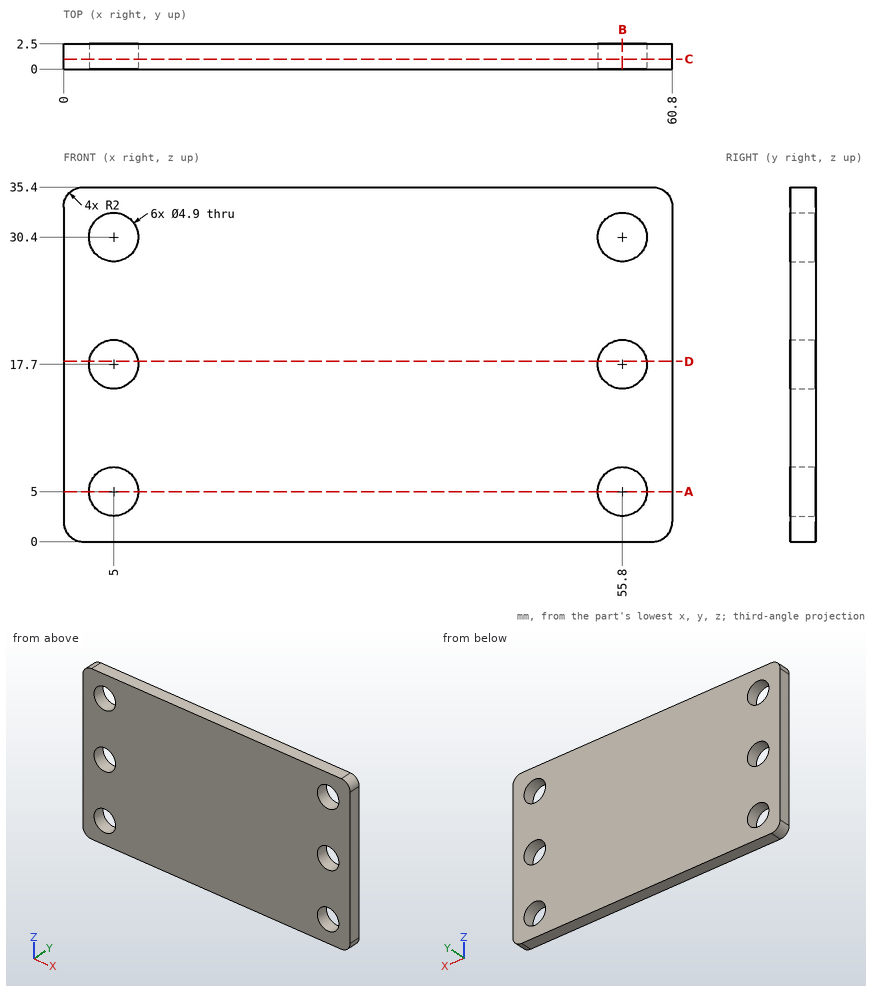
Study the drawing (mm; zero at the part's minimum x, y, z) and answer. Give positions to 0.01 mm unless a question says otherwise; leave off trailing zeros. Write each loop counter-clockwise with the first axis right and the second up, starting at its lowest first coordinate (ties: lowest second). Pieces come first, ordered by that corner, then holes. Notation, with made-up numbers: (75, 22.5) -> (94, 22.5) arc R19 ccw to (94, 58.5) -> close; hole circle Ø1 at (-2.5, 17.25). An arc over 180 degrees is marked (long way). Write item = value, one per line.
Q1. Section B-B on x = 55.8 is taken. Determine the outline of the cut face in (y, z), and give its area (4 significant figures).
Computed values:
outline = (0, 0) -> (2.5, 0) -> (2.5, 2.55) -> (0, 2.55) -> close; (0, 7.45) -> (2.5, 7.45) -> (2.5, 15.25) -> (0, 15.25) -> close; (0, 20.15) -> (2.5, 20.15) -> (2.5, 27.95) -> (0, 27.95) -> close; (0, 32.85) -> (2.5, 32.85) -> (2.5, 35.4) -> (0, 35.4) -> close
area = 51.75 mm^2
Q2. Section C-C on y = 1 is taken. Determine the outline of the cut face in (x, z), and give its area (3 significant figures).
Computed values:
outline = (0, 2) arc R2 ccw to (2, 0) -> (58.8, 0) arc R2 ccw to (60.8, 2) -> (60.8, 33.4) arc R2 ccw to (58.8, 35.4) -> (2, 35.4) arc R2 ccw to (0, 33.4) -> close; hole circle Ø4.9 at (5, 5); hole circle Ø4.9 at (5, 17.7); hole circle Ø4.9 at (5, 30.4); hole circle Ø4.9 at (55.8, 5); hole circle Ø4.9 at (55.8, 17.7); hole circle Ø4.9 at (55.8, 30.4)
area = 2,040 mm^2
Q3. Consider line 1 along Z through (x, y) = (55.8, 0.55); line 2 along X through (y, z) = (1.8, 17.7); line 3 along Z through (x, y) = (58, 1.15). Determine where each line is inside the solid, lowest interval first.
Computed values:
line_1 = 0 to 2.55, 7.45 to 15.25, 20.15 to 27.95, 32.85 to 35.4
line_2 = 0 to 2.55, 7.45 to 53.35, 58.25 to 60.8
line_3 = 0 to 3.92, 6.08 to 16.62, 18.78 to 29.32, 31.48 to 35.4
Q4. Section A-A on z = 5 is taken. Determine the outline of the cut face in (x, y).
Computed values:
outline = (0, 0) -> (2.55, 0) -> (2.55, 2.5) -> (0, 2.5) -> close; (7.45, 0) -> (53.35, 0) -> (53.35, 2.5) -> (7.45, 2.5) -> close; (58.25, 0) -> (60.8, 0) -> (60.8, 2.5) -> (58.25, 2.5) -> close
Q5. Section D-D on z = 18 is taken. Determine the outline of the cut face in (x, y).
Computed values:
outline = (0, 0) -> (2.57, 0) -> (2.57, 2.5) -> (0, 2.5) -> close; (7.43, 0) -> (53.37, 0) -> (53.37, 2.5) -> (7.43, 2.5) -> close; (58.23, 0) -> (60.8, 0) -> (60.8, 2.5) -> (58.23, 2.5) -> close
